Design review of the part built by this model. Coordinates are the model's own, in mm. A direction names the side the tool comes from. Round coordinates to 2 decimals unless told otherwise and drop trailing zeros. Loops run counter-clockwise (first coordinate to the right, second up) from the corner with the lowest first, then second, coordinate; pieces in that order, holes last. Notation, with made-up numbers: (-14.75, 15) -> (29.25, 15) arc R34 ccw to (29.25, 53) -> close; hole circle Ø4 at (13.5, 75.25). An arc over 180 degrees is marked (long way). Write each question's results on one line, items separated by ' | '. Start each with the question number.
from build123d import *

# Parameters (mm, degrees)
F0_W     = 2
F0_H     = 4
F0_H_2   = 2.8740456328
F1_DEPTH = 15
F2_R     = 0.99999
F0_W_2   = 26
F0_H_3   = 7
F3_DEPTH = 2


# Not quite as in the source:
# - a fillet or chamfer is up to 0.001 mm smaller than in the source, because OpenCascade refuses the exact size


with BuildPart() as f1:
    # F0 (on Top) → F1 (new body)
    with BuildSketch(Plane.XY):
        Polygon((14.5, 18.75), (-14.5, 18.75), (-14.5, 13.8759543672), (-14.5, 9.8759543672), (-14.5, -18.75), (14.5, -18.75), (14.5, 9.8759543672), (14.5, 13.8759543672), align=None)
        Polygon((-13, 4.7144976147), (-13, 17.25), (13, 17.25), (13, 4.7144976147), (13, -2.2855023853), (13, -17.25), (-13, -17.25), (-13, -2.2855023853), align=None, mode=Mode.SUBTRACT)
        with Locations((-15.5, 11.8759543672)):
            Rectangle(F0_W, F0_H)
        Polygon((-16.5, 9.8759543672), (-16.5, 13.8759543672), (-16.5, 29.8609879265), (-19.8, 24.85), (-18, 24.85), (-18, 12.75), (-18, 9.8759543672), align=None)
        with Locations((15.5, 11.8759543672)):
            Rectangle(F0_W, F0_H)
        Polygon((16.5, 29.8609879265), (16.5, 13.8759543672), (16.5, 9.8759543672), (18, 9.8759543672), (18, 12.75), (18, 24.85), (19.8, 24.85), align=None)
        with Locations((-19, 11.3129771836)):
            Rectangle(F0_W, F0_H_2)
        with Locations((19, 11.3129771836)):
            Rectangle(F0_W, F0_H_2)
    extrude(amount=F1_DEPTH)

    # F2 (radius 1 in the source; OpenCascade refuses exactly that, so slightly less here)
    f2_edges = [f1.edges().sort_by_distance(p)[0] for p in [
        (-14.5, 18.75, 7.5),
        (-20, 9.875954, 7.5),
        (14.5, 18.75, 7.5),
        (20, 9.875954, 7.5),
        (-13, 17.25, 7.5),
        (14.5, 9.875954, 7.5),
        (14.5, -18.75, 7.5),
        (-14.5, -18.75, 7.5),
        (-13, -17.25, 7.5),
        (13, 17.25, 7.5),
        (13, -17.25, 7.5),
        (-14.5, 13.875954, 7.5),
        (16.5, 13.875954, 7.5),
        (-16.5, 13.875954, 7.5),
        (14.5, 13.875954, 7.5),
        (-16.5, 29.860988, 7.5),
        (16.5, 29.860988, 7.5),
    ]]
    fillet(f2_edges, radius=F2_R)

    # F0 (on Top) → F3 (join)
    with BuildSketch(Plane.XY):
        with Locations((0, 1.2144976147)):
            Rectangle(F0_W_2, F0_H_3)
    extrude(amount=F3_DEPTH)


solid = f1.part
1) Insertion check: pin 1 (4.5 mm diameter, centred on y = -10.5, z = 4, fed in from +X); pin 2 (3.5 mm diameter, centred on y = 21, z = 7, fed in from -X); pin 3 (6 mm diameter, centred on x = 0.5, z = 2.5, fed in from +Y). Each pin has a flat end and moves straight along its axis. Give the tip position at first contact, or say it passes through.
2) To check wall thickness, follow line 1 (X direction, y = 15.5, z = 4); line 2 (X direction, y = 17.5, z = 4.5); line 3 (X direction, y = -8.5, z = 4). State the ranges of each line that lie inside material, in increasing order. Write a range as from..to.
3) Take a section at C-C (y = 3.5). Write out the cut boundary in (x, z), plus the area to 3 significant figures.
4) For faces 1 (the face through (14.5, -5, 7)), 2 (the face through (-16.2, 14.16, 7.6)), 3 (the face through (-12.715, -16.949, 7.605)), list the 3-axis set-ups (+Z, -Z, +X, -X, +Y, -Y) from which the entire face can be reached by the end or side of a thin tool; tool diameter is ignored.
5) Take a section at A-A (x = -1.5). Write out the cut boundary in (y, z), plus the area to 3 significant figures.
6) The part is to be moulded in two halves that separate along X. For faces 4 (the face through (-13, 0, 7)), 5 (the face through (18, 19, 7)), 6 (the face through (19, 12.75, 7)), say which applies: +X half, -X half, draft (parallel to the pull), parting line (faces both ways), or undercut.
7) Take a section at B-B (y = -12). Write out the cut boundary in (x, z), plus the area to 3 significant figures.
Geometry check:
1) pin 1: stops at x = 14.5 | pin 2: stops at x = -18 | pin 3: stops at y = 18.75
2) line 1: x = -18..-16.5, -14.5..-13, 13..14.5, 16.5..18 | line 2: x = -18..-16.5, -14.5..14.5, 16.5..18 | line 3: x = -14.5..-13, 13..14.5
3) outline: (-14.5, 0) -> (14.5, 0) -> (14.5, 15) -> (13, 15) -> (13, 2) -> (-13, 2) -> (-13, 15) -> (-14.5, 15) -> close | area: 97.0 mm^2
4) face 1: +Z, -Z, +X, -Y | face 2: +Z, -Z, +Y | face 3: +Z, -Z
5) outline: (-18.75, 0) -> (-17.25, 0) -> (-17.25, 15) -> (-18.75, 15) -> close; (-2.29, 0) -> (4.71, 0) -> (4.71, 2) -> (-2.29, 2) -> close; (17.25, 0) -> (18.75, 0) -> (18.75, 15) -> (17.25, 15) -> close | area: 59.0 mm^2
6) face 4: undercut | face 5: +X half | face 6: draft
7) outline: (-14.5, 0) -> (-13, 0) -> (-13, 15) -> (-14.5, 15) -> close; (13, 0) -> (14.5, 0) -> (14.5, 15) -> (13, 15) -> close | area: 45.0 mm^2
